The listing builds one solid part. Answer for the finished solid, in the listing's coordinates (mm). Round coordinates to 2 decimals unless told otherwise and drop trailing zeros. Write each loop counter-clockwise with the first axis right and the second up, starting at its lowest first coordinate (ties: lowest second). Pieces come first, ordered by that corner, then holes. Notation, with made-up numbers: (24, 20.5) - (69, 20.5) arc R23 cw to (69, 50.5) - close; hole circle Ø10 at (37, 78.25). An arc over 180 degrees is marked (long way). Use a Markdown table: item, result. Add a question column.
1) A cutting plane is placed at B-B (y = 15). Give the vertices of the cut face in (x, z).
2) A cutting plane is placed at C-C (x = 18). Give the vertices of the cut face in (y, z), then the cut area to 3 significant figures.
3) Find the intervals of material crossed by probe 1 along X at (y, z) = (16.25, -30); probe 2 along Z at (x, y) = (-6, 1); probe 3 along X at (y, z) = (2.5, -20), in increasing order. Write a range as from..to.
4) A cutting plane is placed at A-A (z = -9.5). Give the vertices of the cut face in (x, y).
Autodesk Inventor part; units mm, degrees
ref_plane "YZ Plane" through (0, 0, 0) normal (1, 0, 0) x (0, 1, 0)
ref_plane "XZ Plane" through (0, 0, 0) normal (0, 1, 0) x (-1, 0, 0)
ref_plane "XY Plane" through (0, 0, 0) normal (0, 0, 1) x (1, 0, 0)
sketch "スケッチ1" plane through (0, 0, 0) normal (0, 1, 0) x (-1, 0, 0)
  line L0 (20.1905, 18.381) -> (-27.8095, 18.381)
  line L1 (-27.8095, 18.381) -> (-27.8095, -38.619)
  line L2 (-27.8095, -38.619) -> (20.1905, -38.619)
  line L3 (20.1905, -38.619) -> (20.1905, 18.381)
  point P0 (0, 0)
  dimension "d0" = 48
  dimension "d1" = 57
extrude "押し出し1" add sketch "スケッチ1" along normal blind 17
fillet "フィレット1" radius 3 12 edges at (27.8095, 17, -10.119) (3.8095, 17, -38.619) (-20.1905, 17, -10.119) (3.8095, 17, 18.381) (-20.1905, 8.5, 18.381) (27.8095, 8.5, 18.381) (3.8095, 0, 18.381) (27.8095, 0, -10.119) (-20.1905, 0, -10.119) (-20.1905, 8.5, -38.619) (27.8095, 8.5, -38.619) (3.8095, 0, -38.619)
sketch "スケッチ2" plane through (0, 17, 0) normal (0, 1, 0) x (1, 0, 0)
  line L0 (18.8095, 10.119) -> (18.8095, 38.619) construction
  line L1 (-17.1905, 38.619) -> (24.8095, 38.619) construction
  line L2 (18.8095, 10.119) -> (18.8095, -18.381) construction
  line L3 (24.8095, -18.381) -> (-17.1905, -18.381) construction
  line L4 (27.8095, -15.381) -> (27.8095, 35.619) construction
  point P0 (0, 0)
  dimension "d5" = 9
hole "穴1" at (18.8095, 17, -10.119) direction (0, -1, 0) diameter 3.4 depth 17
properties part number "batterybox" material "ABS プラスチック"
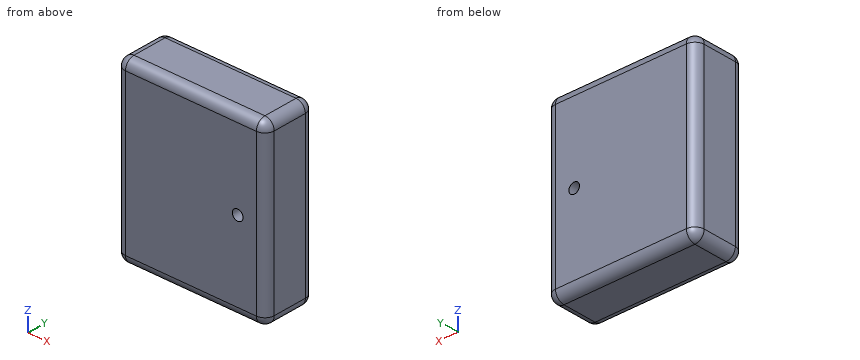
Entries:
| question | item | result |
|---|---|---|
| 1 | outline | (-20.02, -35.62) arc R2.83 ccw to (-17.19, -38.45) - (24.81, -38.45) arc R2.83 ccw to (27.64, -35.62) - (27.64, 15.38) arc R2.83 ccw to (24.81, 18.21) - (-17.19, 18.21) arc R2.83 ccw to (-20.02, 15.38) - close; hole circle Ø3.4 at (18.81, -10.12) |
| 2 | outline | (0, -35.62) arc R3 ccw to (3, -38.62) - (14, -38.62) arc R3 ccw to (17, -35.62) - (17, -11.61) - (0, -11.61) - close; (0, -8.62) - (17, -8.62) - (17, 15.38) arc R3 ccw to (14, 18.38) - (3, 18.38) arc R3 ccw to (0, 15.38) - close |
| 2 | area | 910 mm² |
| 3 | probe 1 | x = -19.17..26.79 |
| 3 | probe 2 | z = -37.86..17.62 |
| 3 | probe 3 | x = -20.15..27.77 |
| 4 | outline | (-20.19, 3) arc R3 ccw to (-17.19, 0) - (17.23, 0) - (17.23, 17) - (-17.19, 17) arc R3 ccw to (-20.19, 14) - close; (20.39, 0) - (24.81, 0) arc R3 ccw to (27.81, 3) - (27.81, 14) arc R3 ccw to (24.81, 17) - (20.39, 17) - close |
